from build123d import *

# Parameters (mm, degrees)
F1_DEPTH       = 17
F2_DEPTH       = 10
F3_DEPTH       = 5
F4_D           = 6
F4_CSINK_D     = 11.5
F4_CSINK_ANGLE = 90
F5_D           = 4.2


with BuildPart() as f1:
    # F0 (on Top) → F1 (new body)
    with BuildSketch(Plane.XY):
        with BuildLine():
            ThreePointArc((-96.5, 7), (-103.5, 0), (-96.5, -7))
            Line((-96.5, -7), (96.5, -7))
            ThreePointArc((96.5, -7), (103.5, 0), (96.5, 7))
            Line((96.5, 7), (-96.5, 7))
        make_face()
        with BuildLine():
            ThreePointArc((-96.5, -5.5), (-102, 0), (-96.5, 5.5))
            Line((-96.5, 5.5), (96.5, 5.5))
            ThreePointArc((96.5, 5.5), (102, 0), (96.5, -5.5))
            Line((96.5, -5.5), (-96.5, -5.5))
        make_face(mode=Mode.SUBTRACT)
    extrude(amount=-F1_DEPTH)

    # F0 (on Top) → F2 (join)
    with BuildSketch(Plane.XY):
        Polygon((-128, 11.5), (-128, -14.5), (-128, -16.5), (128, -16.5), (128, -14.5), (128, 11.5), align=None)
        with BuildLine():
            Line((96.5, -7), (-96.5, -7))
            ThreePointArc((-96.5, -7), (-103.5, 0), (-96.5, 7))
            Line((-96.5, 7), (96.5, 7))
            ThreePointArc((96.5, 7), (103.5, 0), (96.5, -7))
        make_face(mode=Mode.SUBTRACT)
    extrude(amount=-F2_DEPTH)

    # F0 (on Top) → F3 (join)
    with BuildSketch(Plane.XY):
        with BuildLine():
            Line((125, 18.5), (-125, 18.5))
            ThreePointArc((-125, 18.5), (-132.0710678119, 15.5710678119), (-135, 8.5))
            Line((-135, 8.5), (-135, -9.5))
            ThreePointArc((-135, -9.5), (-133.5355339059, -13.0355339059), (-130, -14.5))
            Line((-130, -14.5), (-128, -14.5))
            Line((-128, -14.5), (-128, 11.5))
            Line((-128, 11.5), (128, 11.5))
            Line((128, 11.5), (128, -14.5))
            Line((128, -14.5), (130, -14.5))
            ThreePointArc((130, -14.5), (133.5355339059, -13.0355339059), (135, -9.5))
            Line((135, -9.5), (135, 8.5))
            ThreePointArc((135, 8.5), (132.0710678119, 15.5710678119), (125, 18.5))
        make_face()
    extrude(amount=-F3_DEPTH)

    # F4 (through all)
    with Locations(Plane.XY):
        with Locations((117.5, 0), (-117.5, 0)):
            CounterSinkHole(F4_D / 2, F4_CSINK_D / 2, counter_sink_angle=F4_CSINK_ANGLE)

    # F5 (through all)
    with Locations(Plane.XY):
        with Locations((-128.15, 10.75), (-38.35, 10.75), (38.35, 10.75), (128.15, 10.75)):
            Hole(F5_D / 2)


solid = f1.part
Model file for the job. Use its own axes, mm. A direction names the side the tool comes from. Give positions to 0.01 mm unless a question says otherwise; leave off trailing zeros. Loops run counter-clockwise (first coordinate to the right, second up) from the corner with the lowest first, then second, coordinate; pieces in that order, holes last.
1) Flat gauge pins, fed straight in: pin 1 Ø1.5 at (x, z) = (37.5, -12) entering from -Y; pin 2 Ø9.5 at (x, y) = (-117.5, 0) entering from +Z; pin 3 Ø0.6 at (x, z) = (129, -1.5) entering from -Y. Where does each tip first touch, or does it go through?
2) Pull direction Y, two halves, no side cores. Call faces 4 (the cylindrical face through (-133.57, -13, -2.46)), 5 (the cylindrical face through (103.5, -0.15, -13.45)), 6 (the cylindrical face through (-39.319, 8.887, -5.07)): +Y half, -Y half, draft (parallel to the pull), parting line (faces both ways), or undercut.
3) Saw through at B-B (x = 117.5). Write the cut outline in (y, z), plus the area to 3 significant figures.
4) Wall check: line 1 (X direction, y = 10, z = -9.25); line 2 (Y direction, x = 24, z = -4.75); line 3 (Y direction, x = -58.5, z = -12.25). Give the ranges that are in metal, low to high.
5) Tool access for faces 1 (the flat face through (84, 11.5, -7)), 2 (the flat face through (-1, -7, -13)), 3 (the cylindrical face through (-103.5, 0.15, -13.45)): list every direction of +Z, -Z, +X, -X, +Y, -Y with a clear straight run to the whole face (end or side of a thin tool).
6) Saw through at A-A (x = -8.5). Write the cut outline in (y, z).
Answer block:
1. pin 1: stops at y = -7
1. pin 2: stops at z = -1
1. pin 3: stops at y = -14.5
2. face 4: -Y half
2. face 5: parting line
2. face 6: undercut
3. outline: (-16.5, -10) - (-3, -10) - (-3, -2.75) - (-5.75, 0) - (-16.5, 0) - close; (3, -10) - (11.5, -10) - (11.5, -5) - (18.5, -5) - (18.5, 0) - (5.75, 0) - (3, -2.75) - close
3. area: 247 mm2
4. line 1: x = -126.19 to -40.31, -36.39 to 36.39, 40.31 to 126.19
4. line 2: y = -16.5 to -5.5, 5.5 to 18.5
4. line 3: y = -7 to -5.5, 5.5 to 7
5. face 1: -Z, +X, -X, +Y
5. face 2: -Z, +X, -X, -Y
5. face 3: -Z, -X
6. outline: (-16.5, -10) - (-7, -10) - (-7, -17) - (-5.5, -17) - (-5.5, 0) - (-16.5, 0) - close; (5.5, -17) - (7, -17) - (7, -10) - (11.5, -10) - (11.5, -5) - (18.5, -5) - (18.5, 0) - (5.5, 0) - close
